Could you check a few things on this model? Use its own coordinates, in mm. Face numbers are marked on the shaded views. A direction names the side the tool comes from. Coordinates: 2 decimals unless noted, no trailing zeros. Loops run counter-clockwise (first coordinate to the right, second up) from the corner with the lowest first, then second, coordinate; pieces in that order, holes last. Notation, with made-up numbers: (41.5, -23.5) - (58.5, -23.5) arc R21 cw to (58.5, -19.5) - close; hole circle Ø1 at (-0.5, 36.5). An arc over 180 degrees is marked (long way). One line per item, written item: value. Start each with the question number.
(1) I'm going to push flat-ended pins straight in: P1, Ø1.5, axis at y = 22.5, z = -0.5, coming from the +X side; P2, Ø0.6, axis at x = 24.5, z = -1, coming from the -Y side. Where does each tip first touch, or does it pass through?
(2) If we section it at D-D on y = 2: Write out the boundary of the cut face in (x, z).
(3) If we section it at B-B on x = 15.5: Write out the boundary of the cut face in (y, z).
(4) If we mould it in two halves opening along Z, with no side actions, what happens to the marked faces 4, 5 and 6? For each: pulls with the +Z half, pulls with the -Z half, needs draft (parallel to the pull), parting line crosses it, or undercut.
(5) If we section it at A-A on y = 12.5: Count the separate pieces of the cut face and the enclosed holes in it, then the cut area to 4 significant figures.
(6) On a 3-axis mill with a long thin cutter (end or side, diameter ignored), from which of +Z, -Z, +X, -X, +Y, -Y can I reach the whole of each face in a straight line? I mean the marked faces 1, 2 and 3. Say none if no direction works.
(7) If I drill on line 1 along Y through (x, z) = (11, 0); line 2 along X through (y, z) = (5.5, 2), over which ranges is the centre line in solid material (lowest first)? Write a range as from..to.
Autodesk Fusion 360 part; units mm, degrees
sketch "Sketch1" plane through (0, 0, 0) normal (0, 0, 1) x (1, 0, 0)
  line L0 (23, 25) -> (0, 25)
  line L1 (0, 25) -> (0, 0)
  line L2 (0, 0) -> (23, 0)
  line L3 (25, 7.5) -> (25, 17.5)
  line L4 (25, 12.5) -> (0, 12.5) construction
  line L5 (25, 7.5) -> (23, 7.5)
  line L6 (23, 7.5) -> (23, 0)
  line L7 (25, 17.5) -> (23, 17.5)
  line L8 (23, 17.5) -> (23, 25)
  line L9 (21, 23) -> (18.75, 23)
  line L10 (18.75, 23) -> (18.75, 2)
  line L11 (18.75, 2) -> (21, 2)
  line L12 (21, 2) -> (22, 7.5)
  line L13 (22, 17.5) -> (21, 23)
  line L14 (16.25, 17.5) -> (13.75, 17.5)
  line L15 (13.75, 17.5) -> (13.75, 7.5)
  line L16 (13.75, 7.5) -> (16.25, 7.5)
  line L17 (16.25, 7.5) -> (16.25, 17.5)
  line L18 (22, 7.5) -> (22, 17.5)
  point P0 (25, 12.5)
  point P1 (18.75, 12.5)
  point P2 (16.25, 12.5)
  point P3 (22, 12.5)
  dimension "d6" = 2
  dimension "d7" = 1
  dimension "d8" = 2
  dimension "d9" = 10
  dimension "d10" = 25
  dimension "d11" = 2
  dimension "d13" = 2.5
  dimension "d14" = 2.5
  dimension "d24" = 23
  dimension "d25" = 10
  dimension "d26" = 6.25
extrude "Extrude1" add sketch "Sketch1" along normal mid plane 5 contours L0 L1 L2 L3 L5 L6 L7 L8 | L9 L10 L11 L12 L13 L18 | L14 L15 L16 L17
extrude "Extrude2" cut sketch "Sketch1" along normal through all and the other way through all contours L14 L15 L16 L17
pattern_linear "R-Pattern1" count 11 spacing 5 along (-1, 0, 0) of "Extrude2"
mirror "Mirror1" about plane through (0, 25, 0) normal (-1, 0, 0) of bodies 1 merged
equation "unit_size = 25 mm"
equation "wall_thickness = 2 mm"
equation "d6 = wall_thickness"
equation "d24 = unit_size * column_units / 2 - wall_thickness"
equation "d25 = 2 * unit_size / 5"
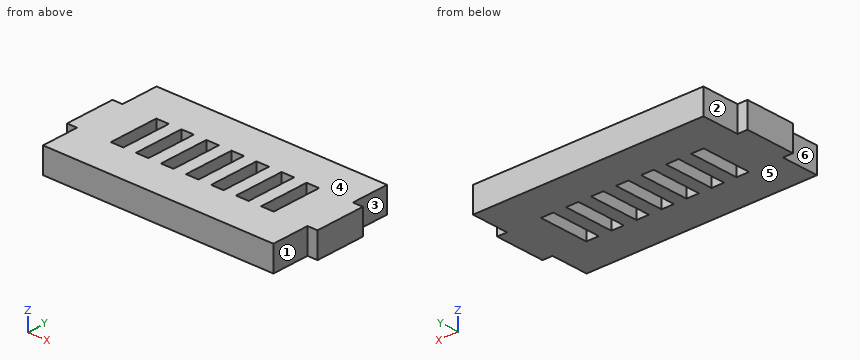
Values:
1. P1: stops at x = 23
1. P2: stops at y = 7.5
2. outline: (-23, -2.5) - (23, -2.5) - (23, 2.5) - (-23, 2.5) - close
3. outline: (0, -2.5) - (7.5, -2.5) - (7.5, 2.5) - (0, 2.5) - close; (17.5, -2.5) - (25, -2.5) - (25, 2.5) - (17.5, 2.5) - close
4. face 4: pulls with the +Z half
4. face 5: pulls with the -Z half
4. face 6: needs draft
5. separate pieces: 8
5. enclosed holes: 0
5. area: 162.5 mm2
6. face 1: +Z, -Z, +X, -Y
6. face 2: +Z, -Z, -X, +Y
6. face 3: +Z, -Z, +X, +Y
7. line 1: y = 0..7.5, 17.5..25
7. line 2: x = -23..23
